Here's how the part is built. I have some questions about the finished solid (model axes, mm). Face numbers are marked on the shaded views. Give positions to 0.01 mm unless a question says otherwise; leave off trailing zeros. Loops run counter-clockwise (first coordinate to the right, second up) from the corner with the lowest first, then second, coordinate; pieces in that order, holes last. Notation, with made-up numbers: (68.5, 84) - (118.5, 84) arc R28 cw to (118.5, 105) - close; hole circle Ø7 at (-24, -12.5). An arc over 180 degrees is marked (long way). One line per item, written item: value. Start each with the question number.
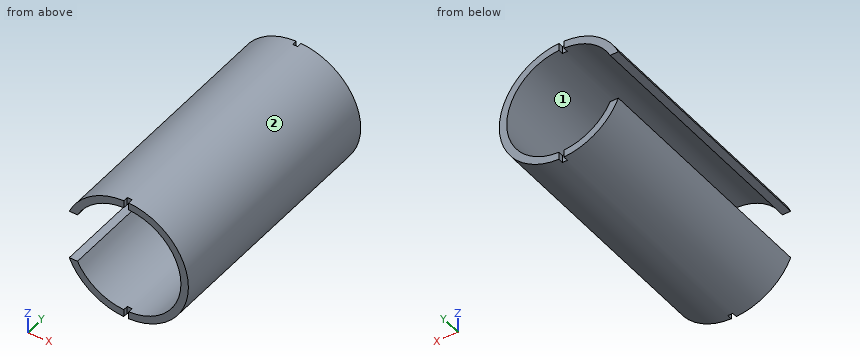
```python
from build123d import *

# Parameters (mm, degrees)
SKETCH_1_R               = 25
SKETCH_1_R_2             = 22
EXTRUDE_1_DEPTH          = 100
CUT_EXTRUDE_1_DEPTH      = 107.066017178
CUT_EXTRUDE_1_DEPTH_BACK = 107.066017178
SKETCH_2_W               = 2
SKETCH_2_H               = 2
CUT_EXTRUDE_4_DEPTH      = 107.066017178
CUT_EXTRUDE_4_DEPTH_BACK = 107.066017178
SKETCH_3_W               = 30.652062969
SKETCH_3_H               = 20


with BuildPart() as part:
    # 草圖1 → 填料-伸長1 (new body)
    with BuildSketch(Plane(origin=(0, 0, 0), x_dir=(1, 0, 0), z_dir=(0, 1, 0))):
        with Locations(Location((0, 0, 0), (0, 0, 270))):
            Circle(SKETCH_1_R)
        with Locations(Location((0, 0, 0), (0, 0, 270))):
            Circle(SKETCH_1_R_2, mode=Mode.SUBTRACT)
    extrude(amount=EXTRUDE_1_DEPTH)

    # 草圖2 → 除料-伸長1 (cut, two sides: drawn at the far end of the back side and taken through both)
    with BuildSketch(Plane.XY.offset(-CUT_EXTRUDE_1_DEPTH_BACK)):
        with Locations((0, 99)):
            Rectangle(SKETCH_2_W, SKETCH_2_H)
        with Locations((0, 1)):
            Rectangle(SKETCH_2_W, SKETCH_2_H)
    extrude(amount=CUT_EXTRUDE_1_DEPTH + CUT_EXTRUDE_1_DEPTH_BACK, mode=Mode.SUBTRACT)

    # 草圖3 → 除料-伸長4 (cut, two sides: drawn at the far end of the back side and taken through both)
    with BuildSketch(Plane(origin=(0, 0, 0), x_dir=(1, 0, 0), z_dir=(0, 1, 0)).offset(-CUT_EXTRUDE_4_DEPTH_BACK)):
        with Locations((-28.265221999, 0)):
            Rectangle(SKETCH_3_W, SKETCH_3_H)
    extrude(amount=CUT_EXTRUDE_4_DEPTH + CUT_EXTRUDE_4_DEPTH_BACK, mode=Mode.SUBTRACT)


solid = part.part
```
(1) If we mould it in two halves opening along Z, with no side actions, what happens to the marked faces 1 and 2? For each: pulls with the +Z half, pulls with the -Z half, needs draft (parallel to the pull), parting line crosses it, or undercut.
(2) Please list where these lines run through material, in increasing order: probe 1 along Z at (x, y) = (0, 38); probe 2 along X at (y, z) = (81, 14); probe 3 along Z at (x, y) = (15, 25.5). Write a range as from..to.
(3) Will these pins go through, and if not, where does the flat tip stop? pin 1 (2 mm diameter, centred on y = 1, z = 24, fed in from -X); pin 2 (2 mm diameter, centred on x = 0, y = 11.5, fed in from -Z); pin 3 (0.6 mm diameter, centred on x = 0, z = 24, fed in from +Y).
(4) If we section it at D-D on z = 0: List the corners of the cut face in (x, y) for me, plus the area to 3 significant figures.
(5) If we section it at B-B on z = -11: List the corners of the cut face in (x, y) for me, plus the area to 3 significant figures.
(6) If we section it at C-C on y = 40: List the corners of the cut face in (x, z) for me, plus the area to 3 significant figures.
(7) If we section it at A-A on x = 0: List the corners of the cut face in (y, z) for me.
Found:
1. face 1: undercut
1. face 2: parting line crosses it
2. probe 1: -25..-22, 22..25
2. probe 2: -20.71..-16.97, 16.97..20.71
2. probe 3: -20..-16.09, 16.09..20
3. pin 1: x = -9.8
3. pin 2: z = -25
3. pin 3: y = 98
4. outline: (22, 0) - (25, 0) - (25, 100) - (22, 100) - close
4. area: 300 mm^2
5. outline: (-22.45, 0) - (-19.05, 0) - (-19.05, 100) - (-22.45, 100) - close; (19.05, 0) - (22.45, 0) - (22.45, 100) - (19.05, 100) - close
5. area: 679 mm^2
6. outline: (-22.91, -10) arc R25 ccw (long way) to (-22.91, 10) - (-19.6, 10) arc R22 cw (long way) to (-19.6, -10) - close
6. area: 381 mm^2
7. outline: (2, -25) - (98, -25) - (98, -22) - (2, -22) - close; (2, 22) - (98, 22) - (98, 25) - (2, 25) - close
